from build123d import *

# Parameters (mm, degrees)
F0_W      = 255
F0_H      = 265
F1_DEPTH  = 5
F3_DEPTH  = 265
F4_R      = 10
F5_DEPTH  = 25
F7_DEPTH  = 25
F9_DEPTH  = 5
F11_DEPTH = 5


with BuildPart() as f1:
    # F0 (on Top) → F1 (new body)
    with BuildSketch(Plane.XY):
        Rectangle(F0_W, F0_H)
    extrude(amount=F1_DEPTH)

    # F2 (on face) → F3 (join)
    with BuildSketch(Plane.XZ.offset(132.5)):
        Polygon((-169.9264068712, 42.4264068712), (-127.5, 0), (-127.5, 5), (-167.4264068712, 44.9264068712), align=None)
        Polygon((127.5, 5), (127.5, 0), (169.9264068712, 42.4264068712), (167.4264068712, 44.9264068712), align=None)
    extrude(amount=-F3_DEPTH)

    # F4 (on face) → F5 (cut)
    with BuildSketch(Plane(origin=(-61.25, 0, -61.25), x_dir=(0, 1, 0), z_dir=(0.7071067812, 0, 0.7071067812))):
        with Locations((0, 150.1561146013)):
            Circle(F4_R)
    extrude(amount=-F5_DEPTH, mode=Mode.SUBTRACT)

    # F6 (on face) → F7 (cut)
    with BuildSketch(Plane(origin=(61.25, 0, -61.25), x_dir=(0, -1, 0), z_dir=(-0.7071067812, 0, 0.7071067812))):
        with BuildLine():
            ThreePointArc((-10, 150.1561146013), (0, 140.1561146013), (10, 150.1561146013))
            Line((10, 150.1561146013), (-10, 150.1561146013))
        make_face()
    extrude(amount=-F7_DEPTH, mode=Mode.SUBTRACT)

    # F8 (on face) → F9 (join)
    with BuildSketch(Plane.XZ.offset(132.5)):
        Polygon((167.4264068712, 44.9264068712), (-167.4264068712, 44.9264068712), (-127.5, 5), (127.5, 5), align=None)
    extrude(amount=-F9_DEPTH)

    # F10 (on face) → F11 (join)
    with BuildSketch(Plane(origin=(0, 132.5, 0), x_dir=(-1, 0, 0), z_dir=(0, 1, 0))):
        Polygon((167.4264068712, 44.9264068712), (-167.4264068712, 44.9264068712), (-127.5, 5), (127.5, 5), align=None)
    extrude(amount=-F11_DEPTH)


solid = f1.part
Geometry: final body of the model. Coordinates: model frame, mm. A direction names the side the tool comes from. Coordinates: 2 decimals unless noted, no trailing zeros. Loops run counter-clockwise (first coordinate to the right, second up) from the corner with the lowest first, then second, coordinate; pieces in that order, holes last. Notation, with made-up numbers: M -37,13.25 L -10,13.25 A33 ccw -10,51.25 Z; hole C -26.75,19.5 d7. An arc over 180 degrees is marked long. One line per item, written item: value. Start each with the question number.
1) Material intervals for L1, parallel to Y at x = 100, z = 8; L2, parallel to Z at x = 22, y = 13; L3, parallel to X at y = -57, z = 23, sorted ascending. Write a range as from..to.
2) Draft query along Y for faces 3 (the flat face through (-2, 2, 0)), 4 (the flat face through (2, 132.5, 23)), 5 (the flat face through (-2, -127.5, 25)). Return one class per face: released by +Y, released by -Y, zero draft, split by the parting line, or undercut.
3) Cut plane B-B (y = 16). Return loops of the section in (x, z).
4) Cut plane C-C (x = -54). Return loops of the section in (y, z), then the cut area to 3 significant figures.
5) Pin query (flat end, axial travel): P1, Ø2, axis at y = -56.5, z = 31.5, coming from the -X side; P2, Ø5, axis at y = 90, z = 6, coming from the +X side; P3, Ø5, axis at y = -45, z = 20, coming from the +X side. Return the tip coordinate at first contact, or that it passes through.
6) Cut plane A-A (z = 14.5). Return loops of the section in (x, y), then the cut area to 3 significant figures.
7) Reachability of faces 1 (the flat face through (-147.2, -1.8, 24.7)), 2 (the flat face through (-2, -132.5, 23)) from +Z, -Z, +X, -X, +Y, -Y: full face, straight path, thin tool, end or side. Return the list, or none.
Evaluation:
1. L1: -132.5..-127.5, 127.5..132.5
1. L2: 0..5
1. L3: -150.5..-145.5, 145.5..150.5
2. face 3: zero draft
2. face 4: released by +Y
2. face 5: undercut
3. outline: M -169.93,42.43 L -127.5,0 L 127.5,0 L 169.93,42.43 L 167.43,44.93 L 127.5,5 L -127.5,5 L -167.43,44.93 Z
4. outline: M -132.5,0 L 132.5,0 L 132.5,44.93 L 127.5,44.93 L 127.5,5 L -127.5,5 L -127.5,44.93 L -132.5,44.93 Z
4. area: 1,720 mm^2
5. P1: x = -160
5. P2: x = 136
5. P3: x = 150
6. outline: M -142,-132.5 L 142,-132.5 L 142,132.5 L -142,132.5 Z; hole M -137,-127.5 L 137,-127.5 L 137,127.5 L -137,127.5 Z
6. area: 5,390 mm^2
7. face 1: +Z
7. face 2: +Z, -Z, +X, -X, -Y
